from build123d import *

# Parameters (mm, degrees)
SKETCH1_W                = 214.089522673
SKETCH1_H                = 271.033566845
BOSS_EXTRUDE1_DEPTH      = 10
SKETCH3_W                = 107.044761337
SKETCH3_H                = 271.033566845
CUT_EXTRUDE1_DEPTH       = 252.253590179
CUT_EXTRUDE2_DEPTH       = 249.55642867
BOSS_EXTRUDE3_DEPTH      = 40
CUT_EXTRUDE3_START       = -165.689856025
CUT_EXTRUDE3_DEPTH       = 205.862728092
CUT_EXTRUDE4_DEPTH       = 250.960593361
CUT_EXTRUDE5_DEPTH       = 250.960593361
CUT_EXTRUDE11_DEPTH      = 252.67545035
SKETCH26_W               = 104.148686
SKETCH26_H               = 11.3
BOSS_EXTRUDE7_DEPTH      = 45
CUT_EXTRUDE12_DEPTH      = 250.816831154
CUT_EXTRUDE13_DEPTH      = 252.67545035
CUT_EXTRUDE14_DEPTH      = 237.436663672
BOSS_EXTRUDE8_DEPTH      = 13.546139965
BOSS_EXTRUDE9_DEPTH      = 30
CUT_EXTRUDE16_DEPTH      = 184.540545695
CUT_EXTRUDE17_DEPTH      = 30
CUT_EXTRUDE17_DEPTH_BACK = 30


with BuildPart() as part:
    # Sketch1 → Boss-Extrude1 (new body)
    with BuildSketch(Plane(origin=(0, 0, 0), x_dir=(1, 0, 0), z_dir=(0, 1, 0))):
        with Locations((-3.148375333, -90.062114546)):
            Rectangle(SKETCH1_W, SKETCH1_H)
    extrude(amount=BOSS_EXTRUDE1_DEPTH)

    # Sketch3 → Cut-Extrude1 (cut, through all)
    with BuildSketch(Plane(origin=(0, 10, 0), x_dir=(1, 0, 0), z_dir=(0, 1, 0))):
        with Locations((-56.670756002, -90.062114546)):
            Rectangle(SKETCH3_W, SKETCH3_H)
    extrude(amount=-CUT_EXTRUDE1_DEPTH, mode=Mode.SUBTRACT)

    # Sketch4 → Cut-Extrude2 (cut, through all)
    with BuildSketch(Plane(origin=(0, 10, 0), x_dir=(1, 0, 0), z_dir=(0, 1, 0))):
        Polygon((103.896386003, -181.239506042), (100.834918545, -173.848469781), (9.996584241, 45.454668877), (103.896386003, 45.454668877), align=None)
    extrude(amount=-CUT_EXTRUDE2_DEPTH, mode=Mode.SUBTRACT)

    # Sketch6 → Boss-Extrude3 (add, along a direction that is not the sketch's normal)
    with BuildSketch(Plane(origin=(0, 10, 0), x_dir=(1, 0, 0), z_dir=(0, 1, 0))):
        Polygon((99.572063218, -170.799667324), (103.896386003, -181.239506042), (-3.148375333, -225.578897968), (-3.148375333, -213.347866105), align=None)
    extrude(amount=BOSS_EXTRUDE3_DEPTH, dir=(-0.2705980500730979, 0.7071067811865489, -0.6532814824381872))

    # Cut-Extrude3: read off the stored shape, not the designer's step
    # Cut-Extrude3 outline → Cut-Extrude3 (cut)
    with BuildSketch(Plane(origin=(0, 0, 0), x_dir=(1, 0, 0), z_dir=(0, 0.6785983445458481, -0.7345095552677544)).offset(CUT_EXTRUDE3_START)):
        Polygon((-3.148375333, -165), (-3.148375333, -152.122604304), (-13.972297336, -155.165042499), (-15, -155.45391393), (-15, -165), align=None)
    extrude(amount=CUT_EXTRUDE3_DEPTH, mode=Mode.SUBTRACT)

    # Sketch8 → Cut-Extrude4 (cut, through all)
    with BuildSketch(Plane(origin=(0, 10, 0), x_dir=(1, 0, 0), z_dir=(0, 1, 0))):
        Polygon((-3.148375333, -225.578897968), (103.896386003, -181.239506042), (103.896386003, -225.578897968), align=None)
    extrude(amount=-CUT_EXTRUDE4_DEPTH, mode=Mode.SUBTRACT)

    # Sketch9 → Cut-Extrude5 (cut, through all)
    with BuildSketch(Plane(origin=(0, 10, 0), x_dir=(1, 0, 0), z_dir=(0, 1, 0))):
        Polygon((-3.148375333, -213.347866105), (99.572063218, -170.799667324), (9.996584241, 45.454668877), (-3.148375333, 45.454668877), align=None)
    extrude(amount=-CUT_EXTRUDE5_DEPTH, mode=Mode.SUBTRACT)

    # Sketch25 → Cut-Extrude11 (cut, through all)
    with BuildSketch(Plane(origin=(24.603270673, 0, -10.191008392), x_dir=(-0.38268343236508967, 0, -0.9238795325112868), z_dir=(0.9238795325112867, 0, -0.3826834323650896))):
        Polygon((-178.918624473, 38.284271247), (-178.918624473, 26.984271247), (-167.618624473, 38.284271247), align=None)
    extrude(amount=-CUT_EXTRUDE11_DEPTH, mode=Mode.SUBTRACT)

    # Sketch26 → Boss-Extrude7 (add)
    with BuildSketch(Plane(origin=(68.469193327, 0, 165.299255136), x_dir=(-0.9238795325112868, 0, 0.3826834323650896), z_dir=(-0.38268343236508956, 0, -0.9238795325112867))):
        with Locations((25.443954722, 32.634271247)):
            Rectangle(SKETCH26_W, SKETCH26_H)
    extrude(amount=BOSS_EXTRUDE7_DEPTH)

    # Sketch27 → Cut-Extrude12 (cut, through all)
    with BuildSketch(Plane.XZ.offset(-26.984271247)):
        Polygon((-3.148375333, 194.964223379), (-3.148375333, 146.256574366), (-20.36912979, 153.389644416), align=None)
    extrude(amount=-CUT_EXTRUDE12_DEPTH, mode=Mode.SUBTRACT)

    # Sketch29 → Cut-Extrude13 (cut, through all)
    with BuildSketch(Plane(origin=(24.603270673, 0, -10.191008392), x_dir=(-0.38268343236508967, 0, -0.9238795325112868), z_dir=(0.9238795325112867, 0, -0.3826834323650896))):
        Polygon((-188.111012628, 17.791883092), (-189.772713564, 19.453584028), (-180.580325409, 28.645972183), (-182.906923537, 30.972570312), (-192.099311693, 21.780182156), (-193.761012628, 23.441883092), (-207.20289572, 10), (-207.20289572, 0), (-195.90289572, 0), (-195.90289572, 10), align=None)
    extrude(amount=-CUT_EXTRUDE13_DEPTH, mode=Mode.SUBTRACT)

    # Sketch31 → Cut-Extrude14 (cut, through all)
    with BuildSketch(Plane(origin=(24.603270673, 0, -10.191008392), x_dir=(-0.38268343236508967, 0, -0.9238795325112868), z_dir=(0.9238795325112867, 0, -0.3826834323650896))):
        Polygon((-133.918624473, 38.284271247), (-165.918624473, 38.284271247), (-165.918624473, 34.284271247), (-178.918624473, 34.284271247), (-178.918624473, 30.984271247), (-165.918624473, 30.984271247), (-165.918624473, 26.984271247), (-133.918624473, 26.984271247), align=None)
    extrude(amount=-CUT_EXTRUDE14_DEPTH, mode=Mode.SUBTRACT)

    # Sketch32 → Boss-Extrude8 (add, along a direction that is not the sketch's normal)
    with BuildSketch(Plane(origin=(29.071379893, -75.967176613, 70.184519615), x_dir=(-0.9626924198811577, -0.19875685341551308, 0.18362738881693294), z_dir=(0.27059805007309423, -0.7071067811865585, 0.6532814824381782))):
        Polygon((33.468379475, -163.963292106), (32.988537984, -163.822749787), (32.063683338, -166.980401064), (33.468379475, -167.391827037), align=None)
    extrude(amount=BOSS_EXTRUDE8_DEPTH, dir=(0, -0.6785983445458523, 0.7345095552677506))

    # Sketch33 → Boss-Extrude9 (add, along a direction that is not the sketch's normal)
    with BuildSketch(Plane(origin=(32.589154544, -85.159564768, 78.677178887), x_dir=(-0.962692419881157, -0.19875685341551325, 0.1836273888169371), z_dir=(0.2705980500730972, -0.7071067811865508, 0.6532814824381854))):
        Polygon((36.642638275, -164.893010983), (24.166759505, -161.238910693), (24.827308404, -158.983655684), (37.122479766, -162.584828001), (37.122479766, -170.910813534), (22.58135596, -166.651816978), (23.241904859, -164.39656197), (35.717783628, -168.05066226), align=None)
    extrude(amount=BOSS_EXTRUDE9_DEPTH, dir=(0, -0.6785983445458483, 0.7345095552677544))

    # Sketch35 → Cut-Extrude16 (cut, through all)
    with BuildSketch(Plane(origin=(39.397813434, 102.95144786, 95.11473552), x_dir=(-0.9626924198811563, 0.19875685341551394, 0.18362738881693996), z_dir=(-0.2705980500730996, -0.7071067811865461, -0.6532814824381894))):
        Polygon((31.899825803, -164.836570859), (46.839732684, -164.836570859), (46.839732684, -169.212368274), (44.194997165, -168.437743175), align=None)
    extrude(amount=-CUT_EXTRUDE16_DEPTH, mode=Mode.SUBTRACT)

    # Sketch37 → Cut-Extrude17 (cut, two sides: drawn at the far end of the back side and taken through both)
    with BuildSketch(Plane(origin=(68.469193327, 0, 165.299255136), x_dir=(-0.9238795325112868, 0, 0.3826834323650897), z_dir=(-0.38268343236508967, 0, -0.9238795325112867)).offset(-CUT_EXTRUDE17_DEPTH_BACK)):
        Polygon((41.018297722, 30.984271247), (41.018297722, 53.15222912), (-28.644246397, 53.15222912), (-28.644246397, 4.37720767), (41.018297722, 4.37720767), align=None)
    extrude(amount=CUT_EXTRUDE17_DEPTH + CUT_EXTRUDE17_DEPTH_BACK, mode=Mode.SUBTRACT)

    # Mirror2: part across plane


with BuildPart() as part_1:
    add(part.part)
    add(part.part.mirror(Plane(origin=(-3.148375333, 0, 225.578897968), x_dir=(0, 0, 1), z_dir=(1, 0, 0))))


solid = part_1.part
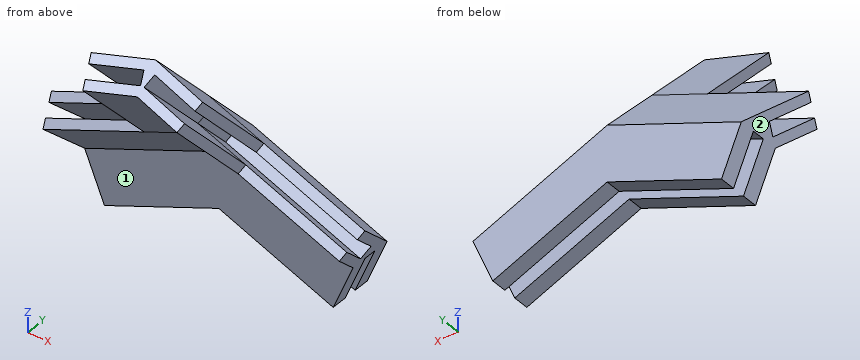
Could you check a few things on this model? Use its own coordinates, in mm. Face numbers are marked on the shaded views. A direction names the side the tool comes from. Round coordinates to 2 decimals unless told otherwise and drop trailing zeros. Loops run counter-clockwise (first coordinate to the right, second up) from the corner with the lowest first, then second, coordinate; pieces in that order, holes last. Notation, with made-up numbers: (64.25, -25.5) - (69.25, -25.5) arc R19 ccw to (69.25, -16.5) - close; hole circle Ø2 at (78.25, -27). An arc over 180 degrees is marked (long way). Write item = value, one per line.
1) Imagine slicing it at D-D (x = -9). Please give me the cut outline in (y, z).
Computed:
outline = (-1.33, 223.19) - (26.98, 192.54) - (26.98, 178.47) - (30.98, 178.47) - (30.98, 192.54) - (34.28, 192.54) - (34.28, 178.47) - (38.28, 178.47) - (38.28, 192.54) - (4.77, 228.82) - (2.97, 227.16) - (30.97, 196.86) - (28.65, 194.34) - (0.46, 224.84) - close
2) Imagine slicing it at C-C (y = 8.5). Please give me the cut outline in (x, z).
Computed:
outline = (-17.15, 221.4) - (-16.51, 218.07) - (-4.5, 223.05) - (-3.61, 218.38) - (-15.62, 213.4) - (-14.98, 210.07) - (-3.15, 214.97) - (8.69, 210.07) - (9.32, 213.4) - (-2.69, 218.38) - (-1.8, 223.05) - (10.21, 218.07) - (10.85, 221.4) - (-3.15, 227.2) - close
3) Imagine slicing it at B-B (z = 186.5). Please give me the cut outline in (x, y), and give its area (3 significant figures).
Computed:
outline = (-39.15, 21.03) - (-23.58, 26.98) - (17.29, 26.98) - (32.85, 21.03) - (32.85, 24.35) - (21.63, 28.65) - (27.71, 30.97) - (32.85, 29) - (32.85, 32.33) - (17.29, 38.28) - (-23.58, 38.28) - (-39.15, 32.33) - (-39.15, 29) - (-34, 30.97) - (-27.93, 28.65) - (-39.15, 24.35) - close; hole (-23.58, 30.98) - (17.29, 30.98) - (17.29, 34.28) - (-23.58, 34.28) - close
area = 603 mm2
4) I'm going to push flat-ended pins straight in: P1, Ø1.5, axis at x = 28, y = 31, coming from the +Z side; P2, Ø21, axis at x = -18, z = 180, coming from the -Y side; P3, Ø1, axis at x = -11, z = 209.5, coming from the -Y side; P4, Ø4, axis at x = 15.5, z = 207, coming from the -Y side. Where does each tip first touch, or does it pass through?
Computed:
P1 = 190.82
P2 = 24.63
P3 = 10.05
P4 = through
5) On a 3-axis mill with a long thin cutter (end or side, diameter ignored), from which of +Z, -Z, +X, -X, +Y, -Y can I reach the whole of each face in a straight line? I mean the marked faces 1 and 2. Say none if no direction works.
Computed:
face_1 = -Z, -Y
face_2 = -Z, -X, +Y, -Y
6) I need wall thicknesses on line 1 along Y through (x, z) = (1, 187.5); line 2 along Z through (x, y) = (-30, 27.5); line 3 along Y through (x, z) = (-30.5, 189). Which ranges of each line are inside material? Lowest first, please. Write a range as from..to.
Computed:
line_1 = 26.98..30.98, 34.28..38.28
line_2 = 169.77..186.88, 191.92..195.51
line_3 = 22.03..25.35, 30..33.33
7) Imagine slicing it at A-A (z = 178). Please give me the cut outline in (x, y).
Computed:
outline = (-35.63, 26.98) - (-10.13, 26.98) - (-10.13, 30.98) - (-35.63, 30.98) - close; (-35.63, 34.28) - (-10.13, 34.28) - (-10.13, 38.28) - (-35.63, 38.28) - close; (3.84, 26.98) - (29.33, 26.98) - (29.33, 30.98) - (3.84, 30.98) - close; (3.84, 34.28) - (29.33, 34.28) - (29.33, 38.28) - (3.84, 38.28) - close
